```python
from build123d import *

# Parameters (mm, degrees)
BOSS_EXTRUDE1_DEPTH        = 2.5
SKETCH6_W                  = 0.64
SKETCH6_H                  = 0.64
CUT_EXTRUDE1_DEPTH         = 2.5
SKETCH15_W                 = 0.64
SKETCH15_H                 = 0.64
CHAMFER4_SIZE              = 0.12
LPATTERN5_COUNT            = 4
LPATTERN5_PITCH            = 2.5
CHAMFER4_OF_LPATTERN5_SIZE = 0.12


with BuildPart() as part:
    # Sketch4 → Boss-Extrude1 (new body)
    with BuildSketch(Plane(origin=(0, 0, 0), x_dir=(1, 0, 0), z_dir=(0, 1, 0))):
        Polygon((-2.37, -0.9), (-2.37, -0.95), (-2.07, -1.25), (-0.47, -1.25), (-0.17, -0.95), (-0.17, -0.9), (0, -0.9), (0, 0.9), (-0.17, 0.9), (-0.17, 0.95), (-0.47, 1.25), (-2.07, 1.25), (-2.37, 0.95), (-2.37, 0.9), (-2.54, 0.9), (-2.54, -0.9), align=None)
    boss_extrude1 = extrude(amount=BOSS_EXTRUDE1_DEPTH)

    # Sketch6 → Cut-Extrude1 (cut)
    with BuildSketch(Plane.XZ):
        with Locations((-1.27, 0)):
            Rectangle(SKETCH6_W, SKETCH6_H)
        with Locations((1.27, 0)):
            Rectangle(SKETCH6_W, SKETCH6_H)
    extrude(amount=-CUT_EXTRUDE1_DEPTH, mode=Mode.SUBTRACT)

    # Sweep1: sweep along a path in Sketch17
    with BuildLine(Plane(origin=(0, 0, 0), x_dir=(1, 0, 0), z_dir=(0, 0, -1))) as sweep1_path:
        Line((-1.27, 6), (-1.27, -4))
        ThreePointArc((-1.27, -4), (-1.416446609, -4.353553391), (-1.77, -4.5))
        Line((-1.77, -4.5), (-5.52, -4.5))
    # Sketch15 → Sweep1 (sweep)
    with BuildSketch(Plane(origin=(0, -6, 0), x_dir=(1, 0, 0), z_dir=(0, 1, 0))):
        with Locations((-1.27, 0)):
            Rectangle(SKETCH15_W, SKETCH15_H)
    sweep1 = sweep(path=sweep1_path.line)

    # Chamfer4
    chamfer4_edges = [part.edges().sort_by_distance(p)[0] for p in [
        (-0.95, -6, 0),
        (-1.59, -6, 0),
        (-1.27, -6, -0.32),
        (-1.27, -6, 0.32),
        (-5.52, 4.18, 0),
        (-5.52, 4.5, 0.32),
        (-5.52, 4.82, 0),
        (-5.52, 4.5, -0.32),
    ]]
    chamfer(chamfer4_edges, length=CHAMFER4_SIZE)

    # LPattern5: Boss-Extrude1, Sweep1 ×4
    with Locations(*[(0, 0, i * LPATTERN5_PITCH) for i in range(1, LPATTERN5_COUNT)]):
        add(boss_extrude1)
        add(sweep1)

    # Chamfer4 of LPattern5
    chamfer4_of_lpattern5_edges = [part.edges().sort_by_distance(p)[0] for p in [
        (-0.95, -6, 2.5),
        (-1.59, -6, 2.5),
        (-1.27, -6, 2.18),
        (-1.27, -6, 2.82),
        (-5.52, 4.18, 2.5),
        (-5.52, 4.5, 2.82),
        (-5.52, 4.82, 2.5),
        (-5.52, 4.5, 2.18),
        (-0.95, -6, 5),
        (-1.59, -6, 5),
        (-1.27, -6, 4.68),
        (-1.27, -6, 5.32),
        (-5.52, 4.18, 5),
        (-5.52, 4.5, 5.32),
        (-5.52, 4.82, 5),
        (-5.52, 4.5, 4.68),
        (-0.95, -6, 7.5),
        (-1.59, -6, 7.5),
        (-1.27, -6, 7.18),
        (-1.27, -6, 7.82),
        (-5.52, 4.18, 7.5),
        (-5.52, 4.5, 7.82),
        (-5.52, 4.82, 7.5),
        (-5.52, 4.5, 7.18),
    ]]
    chamfer(chamfer4_of_lpattern5_edges, length=CHAMFER4_OF_LPATTERN5_SIZE)


solid = part.part
```
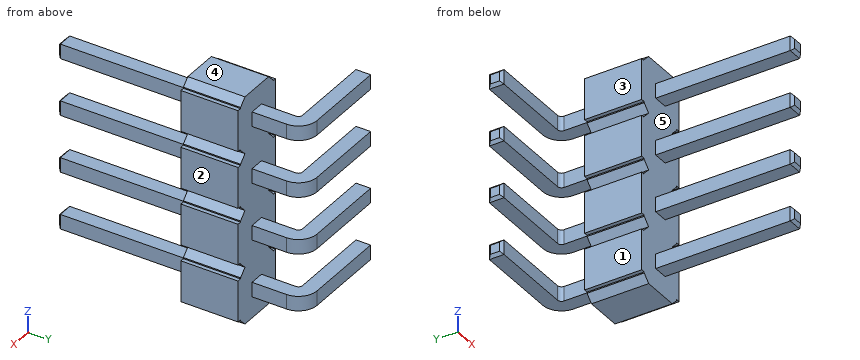
Here's how the part is built. I have some questions about the finished solid (model axes, mm). Face numbers are marked on the shaded views. A direction names the side the tool comes from. Coordinates: 2 decimals unless noted, no trailing zeros. Order: outer loops, then holes, each group sorted by start corner. A loop starts at its lowest first (then second) coordinate and runs counter-clockwise, first axis right, second up.
Item 1: If we section it at B-B, the plane x = -2.75: List the corners of the cut face in (y, z) for me.
Response values:
outline: (4.18, -0.32) - (4.82, -0.32) - (4.82, 0.32) - (4.18, 0.32) - close; (4.18, 2.18) - (4.82, 2.18) - (4.82, 2.82) - (4.18, 2.82) - close; (4.18, 4.68) - (4.82, 4.68) - (4.82, 5.32) - (4.18, 5.32) - close; (4.18, 7.18) - (4.82, 7.18) - (4.82, 7.82) - (4.18, 7.82) - close
Item 2: I'm going to push flat-ended pins straight in: pin 1 Ø1.9 at (x, y) = (-2, 3.5) entering from +Z; pin 2 Ø1 at (x, z) = (-2, 2) entering from -Y; pin 3 Ø1.4 at (y, z) = (1.5, 5) entering from -X. Where does each tip first touch, or does it pass through?
Response values:
pin 1: stops at z = 7.82
pin 2: stops at y = -5.92
pin 3: stops at x = -2.54
Item 3: If we section it at A-A, the plane y = -2.75: List the corners of the cut face in (x, z) for me, then the cut area to 3 significant figures.
Response values:
outline: (-1.59, -0.32) - (-0.95, -0.32) - (-0.95, 0.32) - (-1.59, 0.32) - close; (-1.59, 2.18) - (-0.95, 2.18) - (-0.95, 2.82) - (-1.59, 2.82) - close; (-1.59, 4.68) - (-0.95, 4.68) - (-0.95, 5.32) - (-1.59, 5.32) - close; (-1.59, 7.18) - (-0.95, 7.18) - (-0.95, 7.82) - (-1.59, 7.82) - close
area: 1.64 mm2
Item 4: Which directions (+Z, -Z, +X, -X, +Y, -Y) give clear straight access to the entire face, cutting with the end or side of a thin tool? Please do the marked faces 1 and 2.
Response values:
face 1: +Z, -Z, -X, -Y
face 2: +Z, -Z, +X, +Y, -Y
Item 5: Thinking about a two-plate mould opening in Z: for the marked faces 3, 4 and 5, which applies, pulls with the +Z half, pulls with the -Z half, needs draft (parallel to the pull), parting line crosses it, or undercut?
Response values:
face 3: needs draft
face 4: pulls with the +Z half
face 5: undercut
Item 6: I need wall thicknesses on probe 1 along Y at (x, z) = (-3.35, 2.5); probe 2 along Y at (x, z) = (-2.4, 7.75); probe 3 along X at (y, z) = (4, 7.5). Which ranges of each line are inside material? Lowest first, please.
Response values:
probe 1: y = 4.18 to 4.82
probe 2: y = 0 to 2.5, 4.18 to 4.82
probe 3: x = -1.59 to -0.95
Item 7: If we section it at C-C, the plane z = 1.75: List the corners of the cut face in (x, y) for me, then the cut area to 3 significant figures.
Response values:
outline: (-2.54, 0) - (0, 0) - (0, 2.5) - (-2.54, 2.5) - close
area: 6.35 mm2
